```python
from build123d import *

# Parameters (mm, degrees)
SKETCH1_W           = 8
SKETCH1_H           = 8
BOSS_EXTRUDE1_DEPTH = 55
BOSS_EXTRUDE2_START = 4
BOSS_EXTRUDE2_DEPTH = 14
SKETCH4_R           = 1.25
CUT_EXTRUDE1_DEPTH  = 17.337084372
FILLET1_R           = 2


with BuildPart() as part:
    # Sketch1 → Boss-Extrude1 (new body)
    with BuildSketch(Plane(origin=(0, 0, 0), x_dir=(1, 0, 0), z_dir=(0, 1, 0))):
        with Locations((0, -11)):
            Rectangle(SKETCH1_W, SKETCH1_H)
    extrude(amount=-BOSS_EXTRUDE1_DEPTH)

    # Sketch2 → Boss-Extrude2 (add)
    with BuildSketch(Plane.XY.offset(BOSS_EXTRUDE2_START)):
        with BuildLine():
            Line((-4.720381827, 5.279618173), (-6.61130468, 3.38869532))
            ThreePointArc((-6.61130468, 3.38869532), (0, -2), (6.61130468, 3.38869532))
            Line((6.61130468, 3.38869532), (4.720381827, 5.279618173))
            ThreePointArc((4.720381827, 5.279618173), (4.742589676, 5.015222852), (4.75, 4.75))
            ThreePointArc((4.75, 4.75), (-0.265222852, 0.007410324), (-4.720381827, 5.279618173))
        make_face()
    extrude(amount=BOSS_EXTRUDE2_DEPTH)

    # Sketch4 → Cut-Extrude1 (cut, through all)
    with BuildSketch(Plane(origin=(-5.606601718, -5.606601718, 0), x_dir=(0.707106781, -0.707106781, 0), z_dir=(-0.707106781, -0.707106781, 0))):
        with Locations((-4.342545211, 11)):
            Circle(SKETCH4_R)
    cut_extrude1 = extrude(amount=-CUT_EXTRUDE1_DEPTH, mode=Mode.SUBTRACT)

    # Mirror1: Cut-Extrude1 across plane
    add(cut_extrude1.mirror(Plane(origin=(0, 0, 0), x_dir=(0, 0, 1), z_dir=(1, 0, 0))), mode=Mode.SUBTRACT)

    # Fillet1
    fillet1_edges = [part.edges().sort_by_distance(p)[0] for p in [
        (4, -0.687140793, 11),
        (-4, -0.687140793, 11),
        (0, -2, 15),
        (0, -2, 7),
    ]]
    fillet(fillet1_edges, radius=FILLET1_R)


solid = part.part
```
Source: CAD feature listing. Evaluate the final solid. Frame: model axes, mm. A direction names the side the tool comes from. Coordinates: 2 decimals unless noted, no trailing zeros. Order: outer loops, then holes, each group sorted by start corner. A loop starts at its lowest first (then second) coordinate and runs counter-clockwise, first axis right, second up. Notation, with made-up numbers: (54, 66.25) - (80, 66.25) arc R32 ccw to (80, 95.25) - close; hole circle Ø11 at (65.25, 2.5). An arc over 180 degrees is marked (long way). One line per item, written item: value.
1) Cut plane C-C on y = -26. Output: boundary loops of the cut face in (x, z).
Computed values:
outline: (-4, 7) - (4, 7) - (4, 15) - (-4, 15) - close
2) Mould query, pull axis X, two halves, no side actions, for faces 1 (the face through (-4, -28, 11)), 2 (the face through (6, 4, 11)), 3 (the face through (-5.46, 2.45, 11.05)). Classes: released by +X, released by -X, zero draft, split by the parting line, or undercut.
Computed values:
face 1: released by -X
face 2: released by +X
face 3: undercut
3) Cut plane B-B on z = 8. Output: boundary loops of the cut face in (x, y).
Computed values:
outline: (-6.61, 3.39) arc R6.75 ccw to (-4.63, -0.16) arc R2 cw to (-4, -1.62) - (-4, -55) - (4, -55) - (4, -1.62) arc R2 cw to (4.63, -0.16) arc R6.75 ccw to (6.61, 3.39) - (4.72, 5.28) arc R4.75 cw (long way) to (-4.72, 5.28) - close
4) Ray query, line 1 (Z direction, x = 3.5, y = -30); line 2 (Y direction, x = 0, z = 7.5); line 3 (X direction, y = -9.5, z = 14.5). Return the intervals inside material, ascending. Write a range as [from, to].
Computed values:
line 1: z = [7, 15]
line 2: y = [-55, 0]
line 3: x = [-4, 4]
5) Cut plane A-A on x = 0. Output: boundary loops of the cut face in (y, z), plus the area to 3 significant figures.
Computed values:
outline: (-55, 7) - (-4, 7) arc R2 cw to (-2, 5) - (-2, 4) - (0, 4) - (0, 18) - (-2, 18) - (-2, 17) arc R2 cw to (-4, 15) - (-55, 15) - close
area: 454 mm^2
6) Reachability of faces 4 (the face through (0, -55, 11)), 5 (the face through (4, -28, 11)) from +Z, -Z, +X, -X, +Y, -Y: full face, straight path, thin tool, end or side. Return the list, or none.
Computed values:
face 4: +Z, -Z, +X, -X, -Y
face 5: +Z, -Z, +X, -Y
7) Contact query for flat-ended pins moving along their axis: pin 1 (5 mm diameter, centred on x = -2.5, y = -20, fed in from +Z); pin 2 (6 mm diameter, centred on y = -27, z = 13.5, fed in from -X); pin 3 (1 mm diameter, centred on y = -9, z = 11, fed in from +X). Output: stop coordinate, or through.
Computed values:
pin 1: stops at z = 15
pin 2: stops at x = -4
pin 3: stops at x = 4
